For this review, take the finished solid that the model builds, in its own axes (mm). A direction names the side the tool comes from. Coordinates: 2 decimals unless noted, no trailing zeros. Loops run counter-clockwise (first coordinate to the right, second up) from the corner with the lowest first, then second, coordinate; pieces in that order, holes last.
Autodesk Inventor part; units mm, degrees
ref_plane "YZ Plane" through (0, 0, 0) normal (1, 0, 0) x (0, 1, 0)
ref_plane "XZ Plane" through (0, 0, 0) normal (0, 1, 0) x (-1, 0, 0)
ref_plane "XY Plane" through (0, 0, 0) normal (0, 0, 1) x (1, 0, 0)
sketch "Sketch1" plane through (0, 0, 0) normal (0, 0, 1) x (1, 0, 0)
  line L0 (0, 0) -> (25.4, 0)
  line L1 (25.4, 0) -> (25.4, 50.8)
  line L2 (25.4, 50.8) -> (0, 50.8)
  line L3 (0, 50.8) -> (0, 0)
  dimension "d0" = 25.4
  dimension "d1" = 50.8
extrude "Extrusion1" add sketch "Sketch1" along normal blind 228.6
shell "Shell1" thickness 1.5875 removed faces 2 at (8.4667, 16.9333, 0) at (8.4667, 16.9333, 228.6)
hole "Hole3" at (25.4, 38.1, 12.7) direction (-1, 0, 0) diameter 6.35 end through all
hole "Hole4" at (25.4, 12.7, 12.7) direction (-1, 0, 0) diameter 6.35 end through all
hole "Hole5" at (25.4, 25.4, 177.8) direction (-1, 0, 0) diameter 28.575 end through all
hole "Hole7" at (25.4, 38.1, 215.9) direction (-1, 0, 0) diameter 6.35 end through all
hole "Hole8" at (25.4, 12.7, 215.9) direction (-1, 0, 0) diameter 6.35 end through all
properties part number "Roller Wheel Right Side Support Beam"
Q1. Machinability: for faces 1 (the face through (0.8, 15.5, 11.2)), 2 (the face through (23.812, 25, 113)), which of the approach directions +Z, -Z, +X, -X, +Y, -Y give a long, thin tool a straight path to every point of the face, cutting with its end or side? Answer none if there is none.
Q2. Consider section A-A (z = 177.8). State the section outline as (x, y) points.
Q3. The part is to be moulded in two halves that separate along Y. For faces 3 (the face through (13, 0, 113)), 4 (the face through (0.78, 21.11, 164.17)), 5 (the face through (1, 27, 228.6)), say which applies: +Y half, -Y half, draft (parallel to the pull), parting line (faces both ways), or undercut.
Q4. Wall thickness on probe 1 along Y at (x, z) = (1.25, 215.9) (3 decimals); probe 2 along Y at (x, z) = (12.25, 211); probe 3 along Z at (x, y) = (24.95, 25.4): over which ranges is each line inside the solid? List them lowest first.
Q5. Consider section B-B (y = 25.4). State the section outline as (x, z) points.
Q6. Consider section C-C (x = 8.5). State the section outline as (y, z) points.
Q7. Consider section D-D (y = 44.5). State the section outline as (x, z) points.
Q8. For pin 1 Ø12 at (x, y) = (16.5, 37.5) entering from +Z, flat-tipped, find the tip position at first contact; note if it passes through.
Model answer:
1. face 1: +X, -X
1. face 2: +Z, -Z
2. outline: (0, 0) - (25.4, 0) - (25.4, 11.11) - (23.81, 11.11) - (23.81, 1.59) - (1.59, 1.59) - (1.59, 11.11) - (0, 11.11) - close; (0, 39.69) - (1.59, 39.69) - (1.59, 49.21) - (23.81, 49.21) - (23.81, 39.69) - (25.4, 39.69) - (25.4, 50.8) - (0, 50.8) - close
3. face 3: -Y half
3. face 4: undercut
3. face 5: draft
4. probe 1: y = 0 to 9.525, 15.875 to 34.925, 41.275 to 50.8
4. probe 2: y = 0 to 1.59, 49.21 to 50.8
4. probe 3: z = 0 to 163.51, 192.09 to 228.6
5. outline: (0, 0) - (1.59, 0) - (1.59, 163.51) - (0, 163.51) - close; (0, 192.09) - (1.59, 192.09) - (1.59, 228.6) - (0, 228.6) - close; (23.81, 0) - (25.4, 0) - (25.4, 163.51) - (23.81, 163.51) - close; (23.81, 192.09) - (25.4, 192.09) - (25.4, 228.6) - (23.81, 228.6) - close
6. outline: (0, 0) - (1.59, 0) - (1.59, 228.6) - (0, 228.6) - close; (49.21, 0) - (50.8, 0) - (50.8, 228.6) - (49.21, 228.6) - close
7. outline: (0, 0) - (1.59, 0) - (1.59, 228.6) - (0, 228.6) - close; (23.81, 0) - (25.4, 0) - (25.4, 228.6) - (23.81, 228.6) - close
8. pin 1: passes through
